Design review of the part built by this model. Coordinates are the model's own, in mm. Face numbers are marked on the shaded views. A direction names the side the tool comes from. Round coordinates to 2 decimals unless told otherwise and drop trailing zeros. Write each loop counter-clockwise with the first axis right and the second up, starting at its lowest first coordinate (ties: lowest second). Pieces come first, ordered by that corner, then holes. Notation, with made-up numbers: (-6, 88) -> (29, 88) arc R24 ccw to (29, 112) -> close; hole circle Ø3 at (39, 45). An arc over 180 degrees is marked (long way). Write item = value, one per line. Start each with the question number.
Item 1: Add section B-B, the plane x = 26. State the section outline as (y, z) points.
Item 2: Add section D-D, the plane z = 8.5. State the section outline as (x, y) points, then the cut area to 3 significant figures.
Item 3: Mouldability with a two-part tool opening along Y and no side actions: class the marked faces 1, 2 and 3 as released by +Y, released by -Y, zero draft, split by the parting line, or undercut.
Item 4: Machinability: for the marked faces 4, 5 and 6, which of the approach directions +Z, -Z, +X, -X, +Y, -Y give a long, thin tool a straight path to every point of the face, cutting with its end or side? Answer none if there is none.
Item 5: For pin 1 Ø7 at (x, y) = (21.5, 11) entering from -Z; pin 2 Ø1.5 at (y, z) = (7.5, 6.5) entering from -X; pin 3 Ø1 at (y, z) = (15, 11) entering from -X, all flat-tipped, find the tip position at first contact; note any pin that passes through.
Item 6: Add section C-C, the plane y = 19. State the section outline as (x, z) points, then the cut area to 3 significant figures.
Item 7: To check wall thickness, follow L1, parallel to X at y = 17.75, z = 7.5; L2, parallel to Y at x = 36, z = 9.5; L3, parallel to Z at x = 43.5, y = 18. State the ranges of each line that lie inside material, in increasing order.
from build123d import *

# Parameters (mm, degrees)
BOSS_EXTRUDE1_START = 5
BOSS_EXTRUDE1_DEPTH = 8
BOSS_EXTRUDE2_START = -2
BOSS_EXTRUDE2_DEPTH = 2
FILLET1_R           = 5
FILLET2_R           = 1
FILLET3_R           = 1


with BuildPart() as part:
    # Sketch1 → Boss-Extrude1 (new body)
    with BuildSketch(Plane.XY.offset(BOSS_EXTRUDE1_START)):
        with BuildLine():
            Line((11.509451629, 13.52755518), (11.509451629, 22.52755518))
            ThreePointArc((11.509451629, 22.52755518), (12.534577895, 25.002428914), (15.009451629, 26.02755518))
            Line((15.009451629, 26.02755518), (51, 26.02755518))
            ThreePointArc((51, 26.02755518), (53.474873734, 25.002428914), (54.5, 22.52755518))
            Line((54.5, 22.52755518), (54.5, 1.02755518))
            Line((54.5, 1.02755518), (1.5, 1.02755518))
            Line((1.5, 1.02755518), (0.5, 1.02755518))
            Line((0.5, 1.02755518), (0.5, 0.02755518))
            Line((0.5, 0.02755518), (55.5, 0.02755518))
            Line((55.5, 0.02755518), (55.5, 22.52755518))
            ThreePointArc((55.5, 22.52755518), (54.181980515, 25.709535695), (51, 27.02755518))
            Line((51, 27.02755518), (15.009451629, 27.02755518))
            ThreePointArc((15.009451629, 27.02755518), (11.827471114, 25.709535695), (10.509451629, 22.52755518))
            Line((10.509451629, 22.52755518), (10.509451629, 13.52755518))
            Line((10.509451629, 13.52755518), (11.509451629, 13.52755518))
        make_face()
    extrude(amount=BOSS_EXTRUDE1_DEPTH)

    # Sketch2 → Boss-Extrude2 (add)
    with BuildSketch(Plane.XY.offset(13).offset(BOSS_EXTRUDE2_START)):
        with BuildLine():
            Line((0.5, 5.52755518), (8.509451629, 5.52755518))
            Line((8.509451629, 5.52755518), (8.509451629, 10.52755518))
            Line((8.509451629, 10.52755518), (10.509451629, 10.52755518))
            Line((10.509451629, 10.52755518), (10.509451629, 13.52755518))
            Line((10.509451629, 13.52755518), (10.509451629, 22.52755518))
            ThreePointArc((10.509451629, 22.52755518), (11.827471114, 25.709535695), (15.009451629, 27.02755518))
            Line((15.009451629, 27.02755518), (51, 27.02755518))
            ThreePointArc((51, 27.02755518), (54.181980515, 25.709535695), (55.5, 22.52755518))
            Line((55.5, 22.52755518), (55.5, 0.02755518))
            Line((55.5, 0.02755518), (0.5, 0.02755518))
            Line((0.5, 0.02755518), (0.5, 1.02755518))
            Line((0.5, 1.02755518), (0.5, 5.52755518))
        make_face()
    extrude(amount=BOSS_EXTRUDE2_DEPTH)

    # Fillet1
    fillet1_edges = [part.edges().sort_by_distance(p)[0] for p in [
        (8.509451629, 5.52755518, 12),
    ]]
    fillet(fillet1_edges, radius=FILLET1_R - 0.0001)  # a hair under: the kernel refuses the full size

    # Fillet2
    fillet2_edges = [part.edges().sort_by_distance(p)[0] for p in [
        (10.509451629, 10.52755518, 12),
    ]]
    fillet(fillet2_edges, radius=FILLET2_R)

    # Fillet3
    fillet3_edges = [part.edges().sort_by_distance(p)[0] for p in [
        (11.509451629, 18.02755518, 11),
        (54.5, 11.77755518, 11),
        (27.5, 1.02755518, 11),
        (12.534577895, 25.002428914, 11),
        (33.004725815, 26.02755518, 11),
        (53.474873734, 25.002428914, 11),
    ]]
    fillet(fillet3_edges, radius=FILLET3_R)


solid = part.part
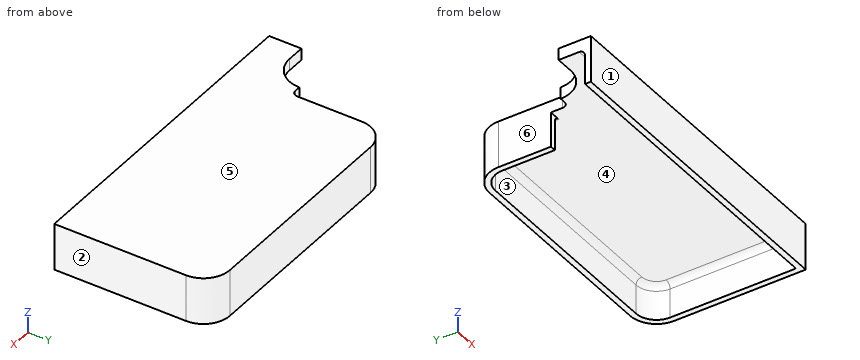
Result set:
q1.outline = (0.03, 5) -> (1.03, 5) -> (1.03, 10) arc R1 cw to (2.03, 11) -> (25.03, 11) arc R1 cw to (26.03, 10) -> (26.03, 5) -> (27.03, 5) -> (27.03, 13) -> (0.03, 13) -> close
q2.outline = (0.5, 0.03) -> (55.5, 0.03) -> (55.5, 22.53) arc R4.5 ccw to (51, 27.03) -> (15.01, 27.03) arc R4.5 ccw to (10.51, 22.53) -> (10.51, 13.53) -> (11.51, 13.53) -> (11.51, 22.53) arc R3.5 cw to (15.01, 26.03) -> (51, 26.03) arc R3.5 cw to (54.5, 22.53) -> (54.5, 1.03) -> (0.5, 1.03) -> close
q2.area = 134 mm²
q3.face_1 = released by -Y
q3.face_2 = zero draft
q3.face_3 = undercut
q4.face_4 = -Z
q4.face_5 = +Z, +X, -X, +Y, -Y
q4.face_6 = +Z, -Z, -X, +Y
q5.pin_1 = 11
q5.pin_2 = 54.5
q5.pin_3 = 10.51
q6.outline = (10.51, 5) -> (11.51, 5) -> (11.51, 10) arc R1 cw to (12.51, 11) -> (53.5, 11) arc R1 cw to (54.5, 10) -> (54.5, 5) -> (55.5, 5) -> (55.5, 13) -> (10.51, 13) -> close
q6.area = 102 mm²
q7.L1 = 10.51 to 11.51, 54.5 to 55.5
q7.L2 = 0.03 to 1.03, 26.03 to 27.03
q7.L3 = 11 to 13
